The listing builds one solid part. Answer for the finished solid, in the listing's coordinates (mm). Face numbers are marked on the shaded views. A direction names the side the tool comes from. Round coordinates to 2 decimals unless told otherwise and drop trailing zeros. Loops run counter-clockwise (first coordinate to the right, second up) from the corner with the lowest first, then second, coordinate; pieces in that order, holes last. Notation, with made-up numbers: (21, 72.5) - (72, 72.5) arc R20 cw to (72, 82.5) - close; hole circle Ø6 at (-32, -2.5). An arc over 180 degrees is marked (long way). Write item = value, one per line. Start each with the question number.
1) Section B-B, the plane y = 0 is taken. Determine the outline of the cut face in (x, z).
2) Straight lines are drawn through the part: line 1 along Y through (x, z) = (0, 3); line 2 along Y through (x, z) = (0, 7.6); line 3 along Z through (x, y) = (-3.5, -1). For each, find the intervals that lie inside material, in ascending order.
3) Section D-D, the plane z = 8.5 is taken. Determine the outline of the cut face in (x, y), and give its area (3 significant figures).
4) Section C-C, the plane x = 0 is taken. Determine the outline of the cut face in (y, z), and give its area (3 significant figures).
5) Given pin 1 Ø2 at (x, z) = (2, 1.5) entering from +Y; pin 2 Ø2.5 at (x, y) = (0, 0) entering from -Z; pin 3 Ø2 at (x, z) = (-3.5, 9.5) entering from -Y; pin 4 Ø0.8 at (x, y) = (1, 1) entering from +Z, each flat-ended and moving along its own axis, determine where each tip first touches the part or whether it passes through.
6) For a pull along Y with two mould halves and no side action, classify the marked faces 1, 2 and 3 as released by +Y, released by -Y, zero draft, split by the parting line, or undercut.
7) A tool of negligible diameter and unlimited length cuts with its end or side. For the marked faces 4, 5 and 6, from which of +Z, -Z, +X, -X, +Y, -Y can it reach the whole face along a straight path? Write none if from no direction.
8) Section A-A, the plane z = 10 is taken. Determine the outline of the cut face in (x, y).
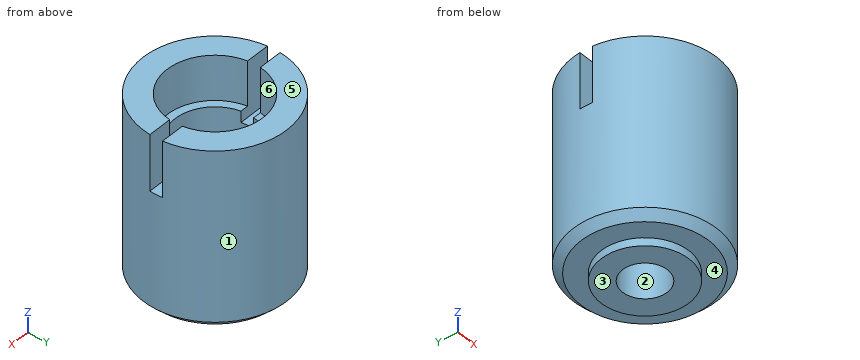
from build123d import *

# Parameters (mm, degrees)
SKETCH1_R           = 2.75
SKETCH1_R_2         = 1.4
BOSS_EXTRUDE1_DEPTH = 0.5
SKETCH2_R           = 4.5
SKETCH2_R_2         = 1.4
BOSS_EXTRUDE2_DEPTH = 6.1
CHAMFER1_SIZE       = 0.5
SKETCH3_R           = 4.5
SKETCH3_R_2         = 2.5
BOSS_EXTRUDE3_DEPTH = 2.2
SKETCH4_R           = 4.5
SKETCH4_R_2         = 3
BOSS_EXTRUDE4_DEPTH = 2.8
SKETCH5_W           = 0.8
SKETCH5_H           = 3.5
CUT_EXTRUDE1_DEPTH  = 4.5


with BuildPart() as part:
    # Sketch1 → Boss-Extrude1 (new body)
    with BuildSketch(Plane(origin=(0, 0, 0), x_dir=(0, 1, 0), z_dir=(0, 0, 1))):
        with Locations(Location((0, 0, 0), (0, 0, 270))):
            Circle(SKETCH1_R)
        with Locations(Location((0, 0, 0), (0, 0, 270))):
            Circle(SKETCH1_R_2, mode=Mode.SUBTRACT)
    extrude(amount=BOSS_EXTRUDE1_DEPTH)

    # Sketch2 → Boss-Extrude2 (add)
    with BuildSketch(Plane.XY.offset(0.5)):
        Circle(SKETCH2_R)
        Circle(SKETCH2_R_2, mode=Mode.SUBTRACT)
    extrude(amount=BOSS_EXTRUDE2_DEPTH)

    # Chamfer1
    chamfer1_edges = [part.edges().sort_by_distance(p)[0] for p in [
        (-4.5, 0, 0.5),
    ]]
    chamfer(chamfer1_edges, length=CHAMFER1_SIZE)

    # Sketch3 → Boss-Extrude3 (add)
    with BuildSketch(Plane.XY.offset(6.6)):
        Circle(SKETCH3_R)
        Circle(SKETCH3_R_2, mode=Mode.SUBTRACT)
    extrude(amount=BOSS_EXTRUDE3_DEPTH)

    # Sketch4 → Boss-Extrude4 (add)
    with BuildSketch(Plane.XY.offset(8.8)):
        Circle(SKETCH4_R)
        Circle(SKETCH4_R_2, mode=Mode.SUBTRACT)
    extrude(amount=BOSS_EXTRUDE4_DEPTH)

    # Sketch5 → Cut-Extrude1 (cut, symmetric)
    with BuildSketch(Plane.YZ):
        with Locations((0, 9.85)):
            Rectangle(SKETCH5_W, SKETCH5_H)
    extrude(amount=CUT_EXTRUDE1_DEPTH, both=True, mode=Mode.SUBTRACT)


solid = part.part
Geometry check:
q1.outline = (-4.5, 1) - (-4, 0.5) - (-2.75, 0.5) - (-2.75, 0) - (-1.4, 0) - (-1.4, 6.6) - (-2.5, 6.6) - (-2.5, 8.1) - (-4.5, 8.1) - close; (1.4, 0) - (2.75, 0) - (2.75, 0.5) - (4, 0.5) - (4.5, 1) - (4.5, 8.1) - (2.5, 8.1) - (2.5, 6.6) - (1.4, 6.6) - close
q2.line_1 = -4.5 to -1.4, 1.4 to 4.5
q2.line_2 = -4.5 to -2.5, 2.5 to 4.5
q2.line_3 = 0.5 to 11.6
q3.outline = (-4.48, -0.4) arc R4.5 ccw to (4.48, -0.4) - (2.47, -0.4) arc R2.5 cw to (-2.47, -0.4) - close; (-4.48, 0.4) - (-2.47, 0.4) arc R2.5 cw to (2.47, 0.4) - (4.48, 0.4) arc R4.5 ccw to start
q3.area = 40.8 mm2
q4.outline = (-4.5, 1) - (-4, 0.5) - (-2.75, 0.5) - (-2.75, 0) - (-1.4, 0) - (-1.4, 6.6) - (-2.5, 6.6) - (-2.5, 8.8) - (-3, 8.8) - (-3, 11.6) - (-4.5, 11.6) - close; (1.4, 0) - (2.75, 0) - (2.75, 0.5) - (4, 0.5) - (4.5, 1) - (4.5, 11.6) - (3, 11.6) - (3, 8.8) - (2.5, 8.8) - (2.5, 6.6) - (1.4, 6.6) - close
q4.area = 56.1 mm2
q5.pin_1 = 4.39
q5.pin_2 = through
q5.pin_3 = -3.74
q5.pin_4 = 6.6
q6.face_1 = split by the parting line
q6.face_2 = undercut
q6.face_3 = zero draft
q7.face_4 = -Z
q7.face_5 = +Z, +X, -X, +Y, -Y
q7.face_6 = +Z
q8.outline = (-4.48, -0.4) arc R4.5 ccw to (4.48, -0.4) - (2.97, -0.4) arc R3 cw to (-2.97, -0.4) - close; (-4.48, 0.4) - (-2.97, 0.4) arc R3 cw to (2.97, 0.4) - (4.48, 0.4) arc R4.5 ccw to start
